Part model, mm, in its own coordinate system. Give positions to 0.01 mm unless a question says otherwise; leave off trailing zeros. Write each loop counter-clockwise with the first axis right and the second up, starting at its lowest first coordinate (ties: lowest second). Pieces come first, ordered by that corner, then holes. Notation, with made-up numbers: (22.5, -15) - (55.5, -15) arc R13 cw to (55.5, 8) - close; hole circle Ø11 at (39, 67.5). An arc over 180 degrees is marked (long way). Answer in a Markdown table with one row per item. Add a question column.
1. Drop a flat-ended pin along its axis: pin 1 Ø6.5 at (x, y) = (-100, -50) entering from +Z. Give the stop position or say it passes through.
2. Probe line 1 along Y through (x, z) = (-100, 2.2); line 2 along X through (y, z) = (50, 3); line 3 along X through (y, z) = (-49, 4.25). List the from-to ranges inside material, lowest first.
3. Band-saw the part on B-B on x = -100. Write the cut outline in (y, z).
4. Band-saw the part on A-A on y = -50. Write the cut outline in (x, z).
5. Pull direction Y, two halves, no side cores. Call faces 1 (the flat face through (-2, 75, 3)), 2 (the flat face through (-2, -75, 3)), 3 (the cylindrical face through (-94.505, -0.242, 3.042)), 4 (the flat face through (-125, -1, 3)): released by +Y, released by -Y, zero draft, split by the parting line, or undercut.
```python
from build123d import *

# Parameters (mm, degrees)
F0_W     = 250
F0_H     = 150
F1_DEPTH = 6
F2_D     = 11
F2_DEPTH = 6


with BuildPart() as f1:
    # F0 (on Top) → F1 (new body)
    with BuildSketch(Plane.XY):
        Rectangle(F0_W, F0_H)
    extrude(amount=F1_DEPTH)

    # F2
    with Locations(Plane(origin=(0, 0, 0), x_dir=(1, 0, 0), z_dir=(0, 0, -1))):
        with Locations((-100, 50), (-100, 0), (-100, -50)):
            Hole(F2_D / 2, depth=F2_DEPTH)


solid = f1.part
```
Values:
| question | item | result |
|---|---|---|
| 1 | pin 1 | passes through |
| 2 | line 1 | y = -75 to -55.5, -44.5 to -5.5, 5.5 to 44.5, 55.5 to 75 |
| 2 | line 2 | x = -125 to -105.5, -94.5 to 125 |
| 2 | line 3 | x = -125 to -105.41, -94.59 to 125 |
| 3 | outline | (-75, 0) - (-55.5, 0) - (-55.5, 6) - (-75, 6) - close; (-44.5, 0) - (-5.5, 0) - (-5.5, 6) - (-44.5, 6) - close; (5.5, 0) - (44.5, 0) - (44.5, 6) - (5.5, 6) - close; (55.5, 0) - (75, 0) - (75, 6) - (55.5, 6) - close |
| 4 | outline | (-125, 0) - (-105.5, 0) - (-105.5, 6) - (-125, 6) - close; (-94.5, 0) - (125, 0) - (125, 6) - (-94.5, 6) - close |
| 5 | face 1 | released by +Y |
| 5 | face 2 | released by -Y |
| 5 | face 3 | undercut |
| 5 | face 4 | zero draft |
